Here's the drawing with two shaded views (mm, measured from the low corner). I have some questions. Coordinates: 2 decimals unless noted, no trailing zeros. Write each loop counter-clockwise with the first axis right and the second up, starting at its lowest first coordinate (ties: lowest second). Pieces come first, ordered by that corner, then holes. Notation, with made-up numbers: M -2,-17 L 21,-17 A27 cw 21,9 Z; hole C -3.75,71 d6. An arc over 180 degrees is marked long. Answer as CSV lines item,"result". Start each with the question number.
Item 1: Suppose I cut it at A-A, the plane z = 15. Write out the boundary of the cut face in (x, y) (3 decimals).
Item 2: Suppose I cut it at C-C, the plane x = 7.25. Write out the boundary of the cut face in (y, z), and give its area (3 significant figures).
Item 3: We'd pull the mould along Z, two halves only. Please class the marked faces 1, 2 and 3: +Z half, -Z half, draft (parallel to the pull), parting line (faces both ways), or undercut.
Item 4: If I drill on line 1 along X through (y, z) = (5.5, 15) (3 decimals); line 2 along Y through (x, z) = (13.5, 28.75); line 3 along X through (y, z) = (1.5, 17), over which ranges is the centre line in solid material (lowest first)? Write a range as [from, to].
Item 5: I'm going to push flat-ended pins straight in: P1, Ø5, axis at x = 19.5, z = 7.5, coming from the -Y side; P2, Ø9, axis at x = 15, z = 15, coming from the +Y side; P3, Ø3, axis at y = 4, z = 26.5, coming from the +X side; P4, Ø3, axis at y = 9, z = 5.5, coming from the +X side. Where does each tip first touch, or does it pass through?
Item 6: Suppose I cut it at D-D, the plane y = 6. Write out the boundary of the cut face in (x, z) (3 decimals), and give its area (3 significant figures).
Item 7: Suppose I cut it at B-B, the plane x = 15. Write out the boundary of the cut face in (y, z) (3 decimals), and give its area (3 significant figures).
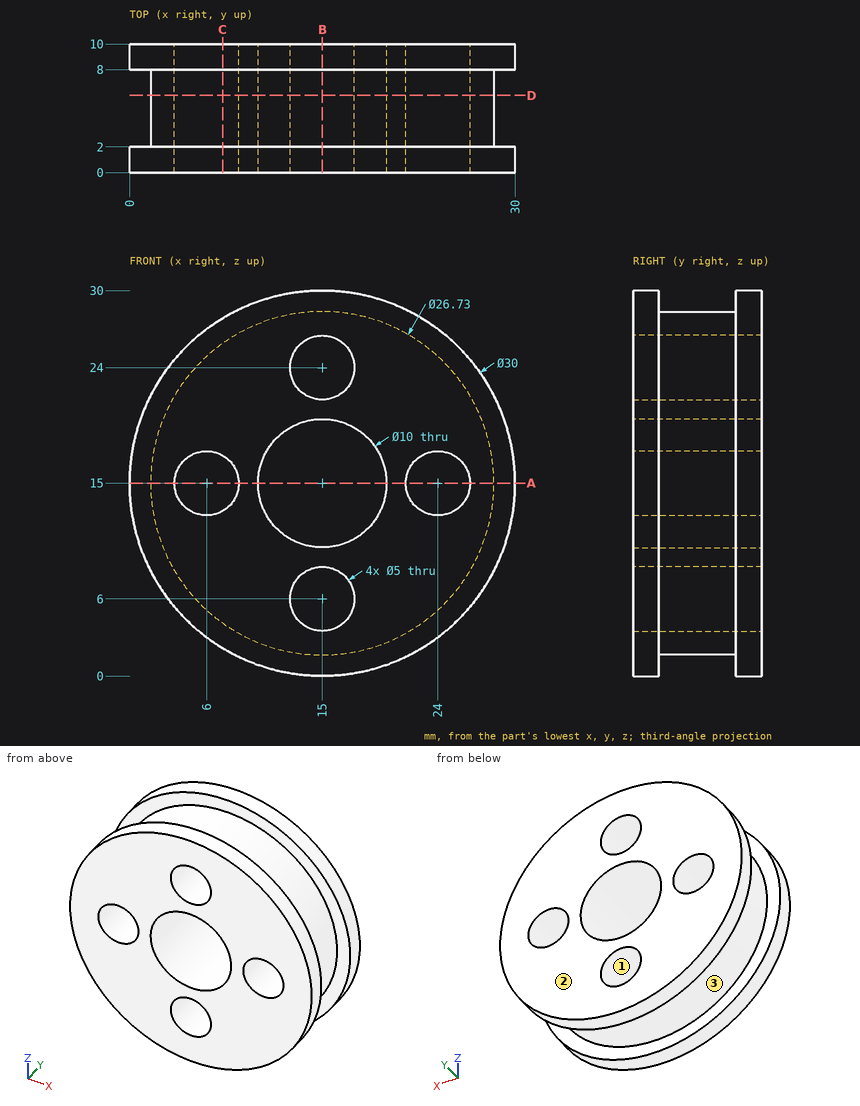
Ans:
1,outline,"M 0,0 L 3.5,0 L 3.5,10 L 0,10 L 0,8 L 1.635,8 L 1.635,2 L 0,2 Z; M 8.5,0 L 10,0 L 10,10 L 8.5,10 Z; M 20,0 L 21.5,0 L 21.5,10 L 20,10 Z; M 26.5,0 L 30,0 L 30,2 L 28.365,2 L 28.365,8 L 30,8 L 30,10 L 26.5,10 Z"
2,outline,"M 0,2.16 L 2,2.16 L 2,4.11 L 8,4.11 L 8,2.16 L 10,2.16 L 10,12.83 L 0,12.83 Z; M 0,17.17 L 10,17.17 L 10,27.84 L 8,27.84 L 8,25.89 L 2,25.89 L 2,27.84 L 0,27.84 Z"
2,area,"190 mm^2"
3,face 1,"undercut"
3,face 2,"draft"
3,face 3,"parting line"
4,line 1,"x = [1.635, 3.5], [8.5, 10], [20, 21.5], [26.5, 28.365]"
4,line 2,"y = [0, 2], [8, 10]"
4,line 3,"x = [0.13, 4.5], [7.5, 10.42], [19.58, 22.5], [25.5, 29.87]"
5,P1,"stops at y = 0"
5,P2,"passes through"
5,P3,"stops at x = 23.87"
5,P4,"stops at x = 27.69"
6,outline,"C 15,15 d26.73; hole C 6,15 d5; hole C 15,15 d10; hole C 15,6 d5; hole C 15,24 d5; hole C 24,15 d5"
6,area,"404 mm^2"
7,outline,"M 0,0 L 2,0 L 2,1.635 L 8,1.635 L 8,0 L 10,0 L 10,3.5 L 0,3.5 Z; M 0,8.5 L 10,8.5 L 10,10 L 0,10 Z; M 0,20 L 10,20 L 10,21.5 L 0,21.5 Z; M 0,26.5 L 10,26.5 L 10,30 L 8,30 L 8,28.365 L 2,28.365 L 2,30 L 0,30 Z"
7,area,"80.4 mm^2"
